Study the drawing (mm; zero at the part's minimum x, y, z) and answer. Round coordinates to 2 decimals unless told otherwise and drop trailing zeros. Write each loop counter-clockwise with the first axis right and the second up, starting at its lowest first coordinate (ties: lowest second). Pieces come first, ordered by that corner, then holes. Notation, with made-up numbers: (-27, -18.5) - (24, -18.5) arc R26 cw to (24, 5.5) - close; hole circle Ø3 at (-13.5, -19). An arc over 180 degrees is marked (long way). Use one line per item in the form item = value. Start each with the question number.
1) The part is cut by section C-C, the plane y = 1.5. Give the vertices of the cut face in (x, z), plus the area to 3 significant figures.
2) The part is cut by section B-B, the plane z = 25.4. Give the vertices of the cut face in (x, y), plus the area to 3 significant figures.
3) The part is cut by section A-A, the plane x = 101.6. Give the vertices of the cut face in (y, z).
4) Consider line 1 along X through (y, z) = (0.95, 25.4); line 2 along Z through (x, y) = (101.6, 1.1); line 3 along X through (y, z) = (0.1, 29). Determine where each line is inside the solid, lowest interval first. Write a range as from..to.
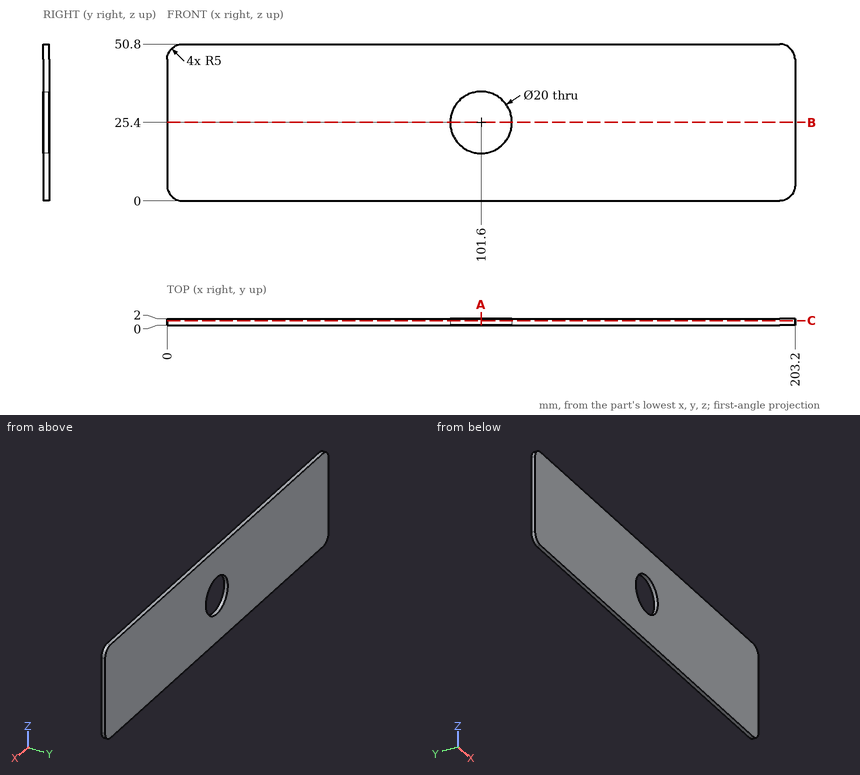
Geometry results:
q1.outline = (0, 5) arc R5 ccw to (5, 0) - (198.2, 0) arc R5 ccw to (203.2, 5) - (203.2, 45.8) arc R5 ccw to (198.2, 50.8) - (5, 50.8) arc R5 ccw to (0, 45.8) - close; hole circle Ø20 at (101.6, 25.4)
q1.area = 9,990 mm2
q2.outline = (0, 0) - (91.6, 0) - (91.6, 2) - (0, 2) - close; (111.6, 0) - (203.2, 0) - (203.2, 2) - (111.6, 2) - close
q2.area = 366 mm2
q3.outline = (0, 0) - (2, 0) - (2, 15.4) - (0, 15.4) - close; (0, 35.4) - (2, 35.4) - (2, 50.8) - (0, 50.8) - close
q4.line_1 = 0..91.6, 111.6..203.2
q4.line_2 = 0..15.4, 35.4..50.8
q4.line_3 = 0..92.27, 110.93..203.2
